from build123d import *

# Parameters (mm, degrees)
SKETCH1_R                                      = 12
SKETCH1_R_2                                    = 3.175
BOSS_EXTRUDE1_DEPTH                            = 3.175
CSK_FOR_6_FLAT_HEAD_MACHINE_SCREW1_D           = 3.7973
CSK_FOR_6_FLAT_HEAD_MACHINE_SCREW1_DEPTH       = 10.973
CSK_FOR_6_FLAT_HEAD_MACHINE_SCREW1_CSINK_D     = 7.0866
CSK_FOR_6_FLAT_HEAD_MACHINE_SCREW1_CSINK_ANGLE = 82
CSK_FOR_6_FLAT_HEAD_MACHINE_SCREW1_TIP         = 1.140824014


with BuildPart() as part:
    # Sketch1 → Boss-Extrude1 (new body)
    with BuildSketch(Plane.XY):
        Circle(SKETCH1_R)
        Circle(SKETCH1_R_2, mode=Mode.SUBTRACT)
    extrude(amount=BOSS_EXTRUDE1_DEPTH)

    # CSK for #6 Flat Head Machine Screw1
    with Locations(Plane(origin=(0, 0, 0), x_dir=(-1, 0, 0), z_dir=(0, 0, -1))):
        with Locations((0, 7.62), (-6.599113577, -3.81), (6.599113577, -3.81)):
            CounterSinkHole(CSK_FOR_6_FLAT_HEAD_MACHINE_SCREW1_D / 2, CSK_FOR_6_FLAT_HEAD_MACHINE_SCREW1_CSINK_D / 2, depth=CSK_FOR_6_FLAT_HEAD_MACHINE_SCREW1_DEPTH, counter_sink_angle=CSK_FOR_6_FLAT_HEAD_MACHINE_SCREW1_CSINK_ANGLE)
            with Locations((0, 0, -(CSK_FOR_6_FLAT_HEAD_MACHINE_SCREW1_DEPTH + CSK_FOR_6_FLAT_HEAD_MACHINE_SCREW1_TIP / 2))):  # 118° drill point
                Cone(0, CSK_FOR_6_FLAT_HEAD_MACHINE_SCREW1_D / 2, CSK_FOR_6_FLAT_HEAD_MACHINE_SCREW1_TIP, mode=Mode.SUBTRACT)


solid = part.part
Geometry check sheet. Reference: the model listing, model coordinates, mm. Give positions to 0.01 mm unless a question says otherwise; leave off trailing zeros. Order: outer loops, then holes, each group sorted by start corner. A loop starts at its lowest first (then second) coordinate and runs counter-clockwise, first axis right, second up.
1) Cross-section at A-A (x = 0). Record the boundary of the cut face in (y, z) (3 decimals).
Results are:
outline: (-12, 0) - (-3.175, 0) - (-3.175, 3.175) - (-12, 3.175) - close; (3.175, 0) - (4.077, 0) - (5.721, 1.892) - (5.721, 3.175) - (3.175, 3.175) - close; (9.519, 1.892) - (11.163, 0) - (12, 0) - (12, 3.175) - (9.519, 3.175) - close
2) Material ranges on probe 1 along Y at (x, z) = (0, 2.95) (3 decimals); probe 2 along X at (y, z) = (-2.25, 0.7); probe 3 along X at (y, z) = (-3.81, 2.4), recorded low to high.
Results are:
probe 1: y = -12 to -3.175, 3.175 to 5.721, 9.519 to 12
probe 2: x = -11.79 to -9.08, -4.11 to -2.24, 2.24 to 4.11, 9.08 to 11.79
probe 3: x = -11.38 to -8.5, -4.7 to 4.7, 8.5 to 11.38
3) Cross-section at D-D (y = 7.62). Record the boundary of the cut face in (x, z) (3 decimals), then the cut area to 3 significant figures.
Results are:
outline: (-9.27, 0) - (-3.543, 0) - (-1.899, 1.892) - (-1.899, 3.175) - (-9.27, 3.175) - close; (1.899, 1.892) - (3.543, 0) - (9.27, 0) - (9.27, 3.175) - (1.899, 3.175) - close
area: 43.7 mm2
4) Gauge pin test, flat ends, axial feed: pin 1 (1 mm diameter, centred on x = 9.5, z = 1, fed in from -Y); pin 2 (1.5 mm diameter, centred on y = -6.5, z = 2, fed in from -X); pin 3 (4.5 mm diameter, centred on x = 0, y = 7.62, fed in from -Z). Record the tip position at first contact, or that the pin passes through.
Results are:
pin 1: stops at y = -7.94
pin 2: stops at x = -10.53
pin 3: stops at z = 1.49
5) Cross-section at B-B (y = -3.81). Record the boundary of the cut face in (x, z) (3 decimals).
Results are:
outline: (-11.379, 0) - (-10.142, 0) - (-8.498, 1.892) - (-8.498, 3.175) - (-11.379, 3.175) - close; (-4.7, 1.892) - (-3.056, 0) - (3.056, 0) - (4.7, 1.892) - (4.7, 3.175) - (-4.7, 3.175) - close; (8.498, 1.892) - (10.142, 0) - (11.379, 0) - (11.379, 3.175) - (8.498, 3.175) - close
6) Cross-section at C-C (z = 2.75). Record the boundary of the cut face in (x, y) (3 decimals).
Results are:
outline: circle Ø24 at (0, 0); hole circle Ø3.797 at (-6.599, -3.81); hole circle Ø6.35 at (0, 0); hole circle Ø3.797 at (0, 7.62); hole circle Ø3.797 at (6.599, -3.81)
7) Draft check along Y on faces 1 (the flat face through (2.5, -2.5, 3.175)), 2 (the cylindrical face through (-11.99, 0.53, 1.57)), 3 (the cylindrical face through (-0.247, 9.502, 2.542)). Enter one of: released by +Y, released by -Y, zero draft, split by the parting line, or undercut.
Results are:
face 1: zero draft
face 2: split by the parting line
face 3: undercut
